Input: part model. Units: mm. Frame: model coordinates. A direction names the side the tool comes from. Give positions to 0.01 mm unless a question says otherwise; leave off trailing zeros. Write each loop counter-clockwise with the first axis right and the second up, starting at its lowest first coordinate (ties: lowest second). Pieces come first, ordered by that corner, then holes. Notation, with made-up numbers: (-10, -20) -> (37, -20) arc R5 ccw to (37, -15) -> close; hole circle Ø8 at (56.5, 86). An arc over 180 degrees is marked (long way). Return JSON: item names as keys, results as strings. Group by question number.
Item 1: Section B-B, the plane y = -30. Return loops of the section in (x, z).
Item 2: Pin query (flat end, axial travel): P1, Ø2.5, axis at x = -16, z = -3, coming from the -Y side; P2, Ø2, axis at y = -10, z = -1, coming from the -X side; P3, Ø1.5, axis at y = -10.5, z = -1, coming from the +X side. Return the tip coordinate at first contact, or that it passes through.
Item 3: Section C-C, the plane x = 19.5. Return loops of the section in (y, z), then the cut area to 3 significant figures.
Item 4: Line query: line 1 (X direction, y = 2, z = -3.5); line 2 (X direction, y = -32, z = -3.95); line 3 (Z direction, x = 2, y = -33.5). Output: solid intervals per line, ascending. Write a range as [from, to].
Item 5: Mould query, pull axis X, two halves, no side actions, for faces 1 (the face through (-17, -32, -3)), 2 (the face through (16.2, -32.7, -5)), 3 (the face through (15, 3, -4)). Classes: released by +X, released by -X, zero draft, split by the parting line, or undercut.
Item 6: Section A-A, the plane x = 0. Return loops of the section in (y, z).
Item 7: Set-up query: faces 4 (the face through (-16, -33.15, -3)), 5 (the face through (6.1, -9, -1)), 6 (the face through (-15, -32, -3)), 7 (the face through (16, -31.65, -3)), 8 (the face through (28.41, -5.49, -0.44)). Return all of +Z, -Z, +X, -X, +Y, -Y with unobstructed straight access to the full face (end or side cutting, diameter ignored); none if empty.
from build123d import *

# Parameters (mm, degrees)
SKETCH_2_R          = 1.7
SKETCH_2_W          = 12.2
SKETCH_2_H          = 4.7
EXTRUDE_1_DEPTH     = 2
SKETCH_3_R          = 3.6
CUT_EXTRUDE_1_DEPTH = 0.9
SKETCH_4_W          = 2
SKETCH_4_H          = 1.5
EXTRUDE_2_DEPTH     = 2
EXTRUDE_3_DEPTH     = 1


with BuildPart() as part:
    # 草图2 → 凸台-拉伸1 (new body)
    with BuildSketch(Plane.XY):
        with BuildLine():
            ThreePointArc((-37.449996405, 0.016409414), (0, -37.45), (37.449996405, 0.016409414))
            ThreePointArc((37.449996405, 0.016409414), (0, 6), (-37.449996405, 0.016409414))
        make_face()
        with Locations((-32.006251973, -5.643565774)):
            Circle(SKETCH_2_R, mode=Mode.SUBTRACT)
        with Locations((32.006251973, -5.643565774)):
            Circle(SKETCH_2_R, mode=Mode.SUBTRACT)
        with Locations((0, -9)):
            Rectangle(SKETCH_2_W, SKETCH_2_H, mode=Mode.SUBTRACT)
    extrude(amount=-EXTRUDE_1_DEPTH)

    # 草图3 → 切除-拉伸1 (cut)
    with BuildSketch(Plane.XY):
        with Locations((-32.006251973, -5.643565774)):
            Circle(SKETCH_3_R)
        with Locations((32.006251973, -5.643565774)):
            Circle(SKETCH_3_R)
    extrude(amount=-CUT_EXTRUDE_1_DEPTH, mode=Mode.SUBTRACT)

    # 草图4 → 凸台-拉伸2 (add)
    with BuildSketch(Plane(origin=(0, 0, -2), x_dir=(-1, 0, 0), z_dir=(0, 0, -1))):
        with Locations((-16, -32.4)):
            Rectangle(SKETCH_4_W, SKETCH_4_H)
        with Locations((16, -32.4)):
            Rectangle(SKETCH_4_W, SKETCH_4_H)
        with BuildLine():
            Line((-18, 1.6), (-18, 4.644461846))
            ThreePointArc((-18, 4.644461846), (-16.002255751, 4.929933515), (-14, 5.181822509))
            Line((-14, 5.181822509), (-14, 1.6))
            Line((-14, 1.6), (-18, 1.6))
        make_face()
        with BuildLine():
            Line((18, 4.644461846), (18, 1.6))
            Line((18, 1.6), (14, 1.6))
            Line((14, 1.6), (14, 5.181822509))
            ThreePointArc((14, 5.181822509), (16.002255751, 4.929933515), (18, 4.644461846))
        make_face()
    extrude(amount=EXTRUDE_2_DEPTH)

    # 草图5 → 凸台-拉伸3 (add)
    with BuildSketch(Plane(origin=(0, 0, -4), x_dir=(-1, 0, 0), z_dir=(0, 0, -1))):
        Polygon((-16.1, -32.5), (-15, -32.5), (-15, -33.15), (-17, -33.15), (-17, -31.65), (-16.1, -31.65), align=None)
        Polygon((16.1, -32.5), (16.1, -31.65), (17, -31.65), (17, -33.15), (15, -33.15), (15, -32.5), align=None)
        with BuildLine():
            Line((-18, 1.6), (-18, 4.644461846))
            ThreePointArc((-18, 4.644461846), (-16.002255751, 4.929933515), (-14, 5.181822509))
            Line((-14, 5.181822509), (-14, 3.7))
            Line((-14, 3.7), (-16.1, 3.7))
            Line((-16.1, 3.7), (-16.1, 1.6))
            Line((-16.1, 1.6), (-18, 1.6))
        make_face()
        with BuildLine():
            Line((14, 3.7), (14, 5.181822509))
            ThreePointArc((14, 5.181822509), (16.002255751, 4.929933515), (18, 4.644461846))
            Line((18, 4.644461846), (18, 1.6))
            Line((18, 1.6), (16.1, 1.6))
            Line((16.1, 1.6), (16.1, 3.7))
            Line((16.1, 3.7), (14, 3.7))
        make_face()
    extrude(amount=EXTRUDE_3_DEPTH)


solid = part.part
Answer below:
{
 "1": {"outline": "(-22.42, -2) -> (22.42, -2) -> (22.42, 0) -> (-22.42, 0) -> close"},
 "2": {"P1": "stops at y = -34.2", "P2": "stops at x = -36.35", "P3": "stops at x = 36.16"},
 "3": {"outline": "(-31.97, -2) -> (4.41, -2) -> (4.41, 0) -> (-31.97, 0) -> close", "area": "72.8 mm2"},
 "4": {"line 1": "x = [-18, -14], [14, 18]", "line 2": "x = [-17, -15], [15, 17]", "line 3": "z = [-2, 0]"},
 "5": {"face 1": "released by -X", "face 2": "zero draft", "face 3": "undercut"},
 "6": {"outline": "(-37.45, -2) -> (-11.35, -2) -> (-11.35, 0) -> (-37.45, 0) -> close; (-6.65, -2) -> (6, -2) -> (6, 0) -> (-6.65, 0) -> close"},
 "7": {"face 4": "-Z, +X, -X, -Y", "face 5": "+Z, -Z", "face 6": "-Z, -Y", "face 7": "-Z, +X, -X", "face 8": "+Z"}
}
